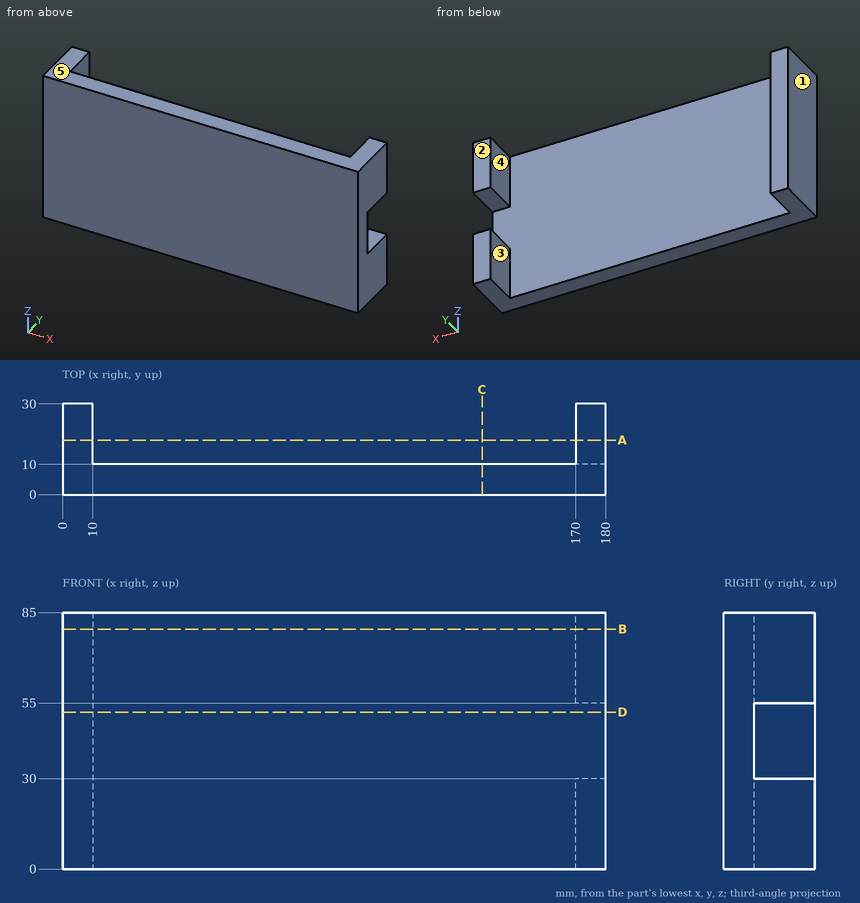
Study the drawing (mm; zero at the part's minimum x, y, z) and answer. A direction names the side the tool comes from. Round coordinates to 2 decimals unless told otherwise and drop trailing zeros. Write each loop counter-clockwise with the first axis right and the second up, starting at its lowest first coordinate (ties: lowest second). Pieces come first, ordered by that corner, then holes. Notation, with made-up numbers: (-21, -8) - (30, -8) arc R20 ccw to (30, 23) - close; hole circle Ø2 at (35.5, 15.25). An arc over 180 degrees is marked (long way). Return JSON: item names as keys, results as strings. Group by question number.
Q1. The part is cut by section D-D on z = 52. Write down the section's boundary in (x, y).
Q2. The part is cut by section C-C on x = 139. Write down the section's boundary in (y, z), then the cut area to 3 significant figures.
Q3. The part is cut by section B-B on z = 79.5. Write down the section's boundary in (x, y), then the cut area to 3 significant figures.
Q4. Find the intervals of material crossed by L1, parallel to X at y = 22, z = 80.5; L2, parallel to Y at x = 65.5, z = 4.5, in increasing order.
Q5. For the marked faces 4 and 5, determine the directions among +Z, -Z, +X, -X, +Y, -Y from which every point of the face is accessible in a straight line to the end or side of a thin tool.
Q6. The part is cut by section A-A on y = 18. Write down the section's boundary in (x, z), then the cut area to 3 significant figures.
Q7. The mould has two halves that part along X. Classify the marked faces 1, 2 and 3: released by +X, released by -X, zero draft, split by the parting line, or undercut.
Q8. Each of these flat-tipped pins is pushed along its axis until it touches: pin 1 Ø6 at (y, z) = (16.5, 40) entering from -X; pin 2 Ø3 at (x, z) = (36, 66.5) entering from +Y. Where does it stop, or does it pass through?
Solved:
{
 "1": {"outline": "(0, 0) - (180, 0) - (180, 10) - (10, 10) - (10, 30) - (0, 30) - close"},
 "2": {"outline": "(0, 0) - (10, 0) - (10, 85) - (0, 85) - close", "area": "850 mm²"},
 "3": {"outline": "(0, 0) - (180, 0) - (180, 30) - (170, 30) - (170, 10) - (10, 10) - (10, 30) - (0, 30) - close", "area": "2,200 mm²"},
 "4": {"L1": "0 to 10, 170 to 180", "L2": "0 to 10"},
 "5": {"face 4": "+Z, -Z, +Y", "face 5": "+Z, +X, -X, +Y, -Y"},
 "6": {"outline": "(0, 0) - (10, 0) - (10, 85) - (0, 85) - close; (170, 0) - (180, 0) - (180, 30) - (170, 30) - close; (170, 55) - (180, 55) - (180, 85) - (170, 85) - close", "area": "1,450 mm²"},
 "7": {"face 1": "released by -X", "face 2": "zero draft", "face 3": "undercut"},
 "8": {"pin 1": "x = 0", "pin 2": "y = 10"}
}
